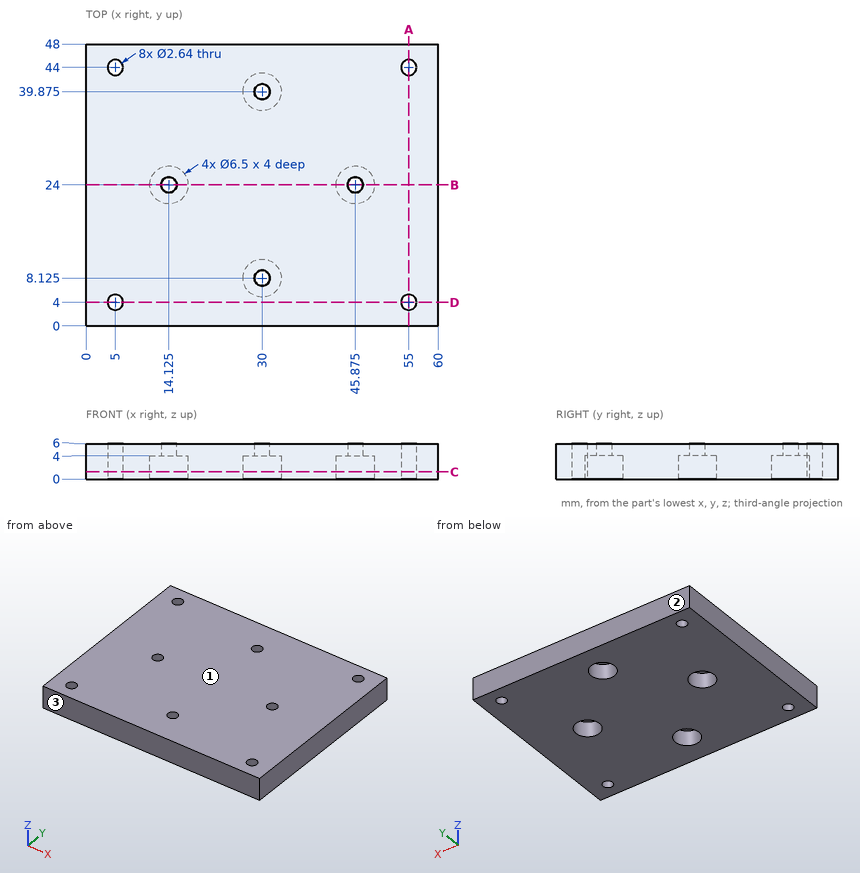
Could you check a few things on this drawing? It's one solid part, dimensions in mm from its lowest x, y, z. Round coordinates to 2 decimals unless told otherwise and drop trailing zeros. Write each loop counter-clockwise with the first axis right and the second up, starting at its lowest first coordinate (ties: lowest second). Pieces come first, ordered by that corner, then holes. Notation, with made-up numbers: (23, 75.5) -> (66, 75.5) arc R28 ccw to (66, 94.5) -> close; hole circle Ø9 at (56.5, -37.5). An arc over 180 degrees is marked (long way). One line per item, written item: value.
1) We'd pull the mould along Y, two halves only. Please class the marked faces 1, 2 and 3: released by +Y, released by -Y, zero draft, split by the parting line, or undercut.
Filled sheet:
face 1: zero draft
face 2: released by +Y
face 3: released by -Y
2) Suppose I cut it at B-B on y = 24. List the corners of the cut face in (x, z) for me (3 decimals).
Filled sheet:
outline: (0, 0) -> (10.875, 0) -> (10.875, 4) -> (12.805, 4) -> (12.805, 6) -> (0, 6) -> close; (15.445, 4) -> (17.375, 4) -> (17.375, 0) -> (42.625, 0) -> (42.625, 4) -> (44.555, 4) -> (44.555, 6) -> (15.445, 6) -> close; (47.195, 4) -> (49.125, 4) -> (49.125, 0) -> (60, 0) -> (60, 6) -> (47.195, 6) -> close
3) Suppose I cut it at C-C on z = 1.2. Give the number of separate pieces and of enclosed holes in the cut face, plus the area to 3 significant figures.
Filled sheet:
separate pieces: 1
enclosed holes: 8
area: 2,730 mm2
4) Suppose I cut it at D-D on y = 4. List the corners of the cut face in (x, z) for me, plus the area to 3 significant figures.
Filled sheet:
outline: (0, 0) -> (3.68, 0) -> (3.68, 6) -> (0, 6) -> close; (6.32, 0) -> (53.68, 0) -> (53.68, 6) -> (6.32, 6) -> close; (56.32, 0) -> (60, 0) -> (60, 6) -> (56.32, 6) -> close
area: 328 mm2
5) If I drill on line 1 (Y direction, x = 55, z = 3.15); line 2 (Y direction, x = 6, z = 4.65); line 3 (X direction, y = 24, z = 5) (3 decimals), over which ranges is the centre line in solid material (lowest first)? Write a range as [from, to].
Filled sheet:
line 1: y = [0, 2.68], [5.32, 42.68], [45.32, 48]
line 2: y = [0, 3.14], [4.86, 43.14], [44.86, 48]
line 3: x = [0, 12.805], [15.445, 44.555], [47.195, 60]
6) I'm going to push flat-ended pins straight in: pin 1 Ø4 at (x, y) = (14.125, 24) entering from -Z; pin 2 Ø1.6 at (x, y) = (5, 4) entering from +Z. Where does each tip first touch, or does it pass through?
Filled sheet:
pin 1: stops at z = 4
pin 2: passes through
7) Suppose I cut it at A-A on x = 55. List the corners of the cut face in (y, z) for me, plus the area to 3 significant figures.
Filled sheet:
outline: (0, 0) -> (2.68, 0) -> (2.68, 6) -> (0, 6) -> close; (5.32, 0) -> (42.68, 0) -> (42.68, 6) -> (5.32, 6) -> close; (45.32, 0) -> (48, 0) -> (48, 6) -> (45.32, 6) -> close
area: 256 mm2
